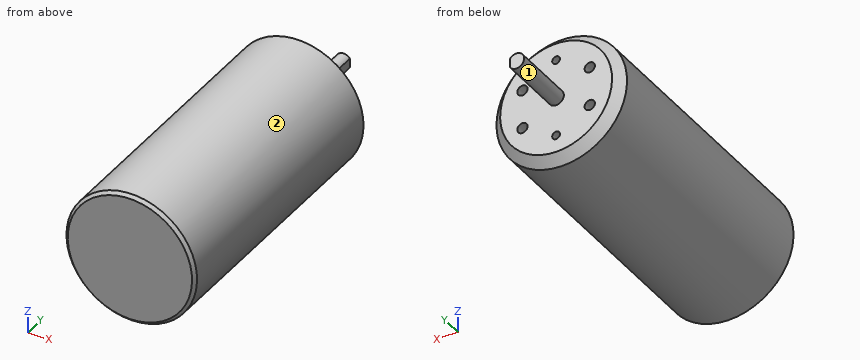
```python
from build123d import *

# Parameters (mm, degrees)
CUT_EXTRUDE1_START              = -17
CUT_EXTRUDE1_DEPTH              = 17
TAP_DRILL_FOR_M3X0_5_TAP1_D     = 2.5
TAP_DRILL_FOR_M3X0_5_TAP1_DEPTH = 9.248924226
TAP_DRILL_FOR_M3X0_5_TAP1_TIP   = 0.751075774
TAP_DRILL_FOR_M4X0_7_TAP1_D     = 3.3
TAP_DRILL_FOR_M4X0_7_TAP1_DEPTH = 9.008579979
TAP_DRILL_FOR_M4X0_7_TAP1_TIP   = 0.991420021
CHAMFER1_SIZE                   = 3
CHAMFER2_SIZE                   = 1


with BuildPart() as part:
    # Sketch1 → Revolve1 (revolve)
    with BuildSketch(Plane.XY, mode=Mode.PRIVATE) as revolve1_sk:
        Polygon((0, 0), (0, 113), (2.5, 113), (2.5, 92), (21, 92), (21, 0), align=None)
    revolve(revolve1_sk.sketch.rotate(Axis((0, 0, 0), (0, 1, 0)), 90), axis=Axis((0, 0, 0), (0, 1, 0)))

    # Sketch2 → Cut-Extrude1 (cut)
    with BuildSketch(Plane(origin=(0, 113, 0), x_dir=(1, 0, 0), z_dir=(0, 1, 0)).offset(CUT_EXTRUDE1_START)):
        with BuildLine():
            Line((2, -1.5), (2, 1.5))
            ThreePointArc((2, 1.5), (2.5, 0), (2, -1.5))
        make_face()
    extrude(amount=CUT_EXTRUDE1_DEPTH, mode=Mode.SUBTRACT)

    # Tap Drill for M3x0.5 Tap1
    with Locations(Plane(origin=(0, 92, 0), x_dir=(1, 0, 0), z_dir=(0, 1, 0))):
        with Locations((0, 12.5), (0, -12.5)):
            Hole(TAP_DRILL_FOR_M3X0_5_TAP1_D / 2, depth=TAP_DRILL_FOR_M3X0_5_TAP1_DEPTH)
            with Locations((0, 0, -(TAP_DRILL_FOR_M3X0_5_TAP1_DEPTH + TAP_DRILL_FOR_M3X0_5_TAP1_TIP / 2))):  # 118° drill point
                Cone(0, TAP_DRILL_FOR_M3X0_5_TAP1_D / 2, TAP_DRILL_FOR_M3X0_5_TAP1_TIP, mode=Mode.SUBTRACT)

    # Tap Drill for M4x0.7 Tap1
    with Locations(Plane(origin=(0, 92, 0), x_dir=(1, 0, 0), z_dir=(0, 1, 0))):
        with Locations((-10.825317547, 6.25), (-10.825317547, -6.25), (10.825317547, -6.25), (10.825317547, 6.25)):
            Hole(TAP_DRILL_FOR_M4X0_7_TAP1_D / 2, depth=TAP_DRILL_FOR_M4X0_7_TAP1_DEPTH)
            with Locations((0, 0, -(TAP_DRILL_FOR_M4X0_7_TAP1_DEPTH + TAP_DRILL_FOR_M4X0_7_TAP1_TIP / 2))):  # 118° drill point
                Cone(0, TAP_DRILL_FOR_M4X0_7_TAP1_D / 2, TAP_DRILL_FOR_M4X0_7_TAP1_TIP, mode=Mode.SUBTRACT)

    # Chamfer1
    chamfer1_edges = [part.edges().sort_by_distance(p)[0] for p in [
        (0, 92, 21),
    ]]
    chamfer(chamfer1_edges, length=CHAMFER1_SIZE)

    # Chamfer2
    chamfer2_edges = [part.edges().sort_by_distance(p)[0] for p in [
        (0, 0, 21),
    ]]
    chamfer(chamfer2_edges, length=CHAMFER2_SIZE)


solid = part.part
```
Could you check a few things on this model? Use its own coordinates, in mm. Face numbers are marked on the shaded views. A direction names the side the tool comes from. Round coordinates to 2 decimals unless told otherwise and drop trailing zeros. Loops run counter-clockwise (first coordinate to the right, second up) from the corner with the lowest first, then second, coordinate; pieces in that order, holes last. Notation, with made-up numbers: (-37, 55.25) - (-20, 55.25) arc R25 ccw to (-20, 67.25) - close; hole circle Ø6 at (40, 59). An arc over 180 degrees is marked (long way). Answer as CSV lines item,"result".
1. For pin 1 Ø5 at (y, z) = (12.5, -11.5) entering from +X; pin 2 Ø2 at (y, z) = (75.5, 3) entering from +X; pin 3 Ø0.5 at (x, z) = (2.5, 0) entering from +Y, each with a flat end and sliding along its axis, tell me the tip position at first contact or that it passes through.
Filled in:
pin 1,"stops at x = 18.97"
pin 2,"stops at x = 20.9"
pin 3,"stops at y = 96"
2. On a 3-axis mill with a long thin cutter (end or side, diameter ignored), from which of +Z, -Z, +X, -X, +Y, -Y can I reach the whole of each face in a straight line? I mean the marked faces 1 and 2. Say none if no direction works.
Filled in:
face 1,"+Y"
face 2,"+Y, -Y"
3. Please list where these lines run through material, in increasing order: line 1 along X through (y, z) = (85, -6); line 2 along X through (y, z) = (86.75, -6.25); line 3 along Y through (x, z) = (-7, -11.5). Write a range as [from, to].
Filled in:
line 1,"x = [-20.12, -12.46], [-9.19, 9.19], [12.46, 20.12]"
line 2,"x = [-20.05, -12.48], [-9.18, 9.18], [12.48, 20.05]"
line 3,"y = [0, 92]"
4. I want a section at A-A on y = 52. List the corners of the cut face in (x, z) for me.
Filled in:
outline,"circle Ø42 at (0, 0)"
